Model file for the job. Use its own axes, mm. Coordinates: 2 decimals unless noted, no trailing zeros. Order: outer loops, then holes, each group sorted by start corner. A loop starts at its lowest first (then second) coordinate and runs counter-clockwise, first axis right, second up. Notation, with made-up numbers: (28, 9.5) -> (79, 9.5) arc R26 ccw to (79, 35.5) -> close; hole circle Ø1 at (-9, 2.5). An arc over 180 degrees is marked (long way). Use CSV: the item, a comma, the result in double quotes. Start each with the question number.
(1) Cut at A-A on y = -17.15. Write the cut outline in (x, z).
(2) Cut at C-C on y = -87. Write the cut outline in (x, z).
(3) Probe L1, parallel to Z at x = -3.7, y = 69.5; L2, parallel to Y at x = -2.2, z = 27; L3, parallel to Z at x = -2.2, y = -94.5. List the from-to ranges inside material, lowest first.
(4) Cut at B-B on x = -0.8. Give the number of separate pieces and of enclosed holes in the cut face, plus the area to 3 significant figures.
(5) Pin check, flat tips, straight feed: pin 1 Ø1.4 at (x, z) = (-3, 56) entering from -Y; pin 2 Ø1.4 at (x, z) = (-1.5, 55) entering from -Y. Stop position of each tip, or through.
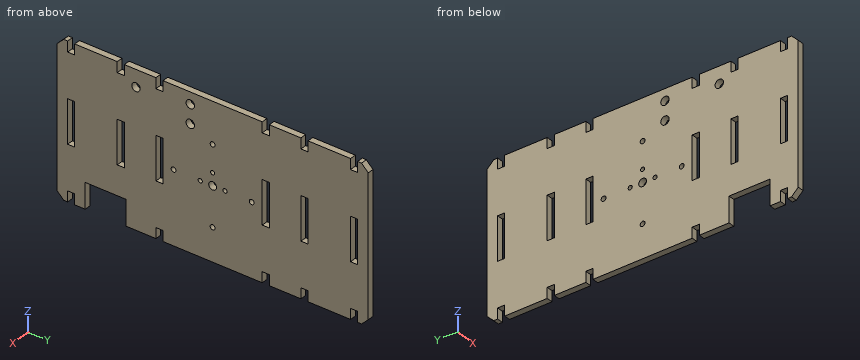
```python
from build123d import *

# Parameters (mm, degrees)
SKETCH1_R           = 1.5875
SKETCH1_R_2         = 3
SKETCH1_R_3         = 3.2385
SKETCH1_R_4         = 1.8669
SKETCH1_W           = 33.02
SKETCH1_H           = 5.461
BOSS_EXTRUDE1_DEPTH = 4.7625
CHAMFER1_SIZE       = 5.08


with BuildPart() as part:
    # Sketch1 → Boss-Extrude1 (new body)
    with BuildSketch(Plane(origin=(0, 0, 0), x_dir=(0, 0, -1), z_dir=(1, 0, 0))):
        Polygon((-58.293, 119.489), (58.293, 119.489), (58.293, 111.361), (50.293, 111.361), (50.293, 105.9), (58.293, 105.9), (58.293, 73.261), (50.293, 73.261), (50.293, 67.8), (58.293, 67.8), (58.293, 43.561), (50.293, 43.561), (50.293, 38.1), (58.293, 38.1), (58.293, -38.1), (50.293, -38.1), (50.293, -43.561), (58.293, -43.561), (58.293, -66.374), (38.857, -66.374), (38.857, -97.87), (58.293, -97.87), (58.293, -105.9), (50.293, -105.9), (50.293, -111.361), (58.293, -111.361), (58.293, -119.489), (-58.293, -119.489), (-58.293, -111.361), (-50.293, -111.361), (-50.293, -105.9), (-58.293, -105.9), (-58.293, -73.261), (-50.293, -73.261), (-50.293, -67.8), (-58.293, -67.8), (-58.293, -43.561), (-50.293, -43.561), (-50.293, -38.1), (-58.293, -38.1), (-58.293, 38.1), (-50.293, 38.1), (-50.293, 43.561), (-58.293, 43.561), (-58.293, 67.8), (-50.293, 67.8), (-50.293, 73.261), (-58.293, 73.261), (-58.293, 105.9), (-50.293, 105.9), (-50.293, 111.361), (-58.293, 111.361), align=None)
        with Locations((3, 9.519071488)):
            Circle(SKETCH1_R, mode=Mode.SUBTRACT)
        with Locations((-6.519071488, 0)):
            Circle(SKETCH1_R, mode=Mode.SUBTRACT)
        with Locations((3, -9.519071488)):
            Circle(SKETCH1_R, mode=Mode.SUBTRACT)
        with Locations((3, 0)):
            Circle(SKETCH1_R_2, mode=Mode.SUBTRACT)
        with Locations((-35.174, -17.15)):
            Circle(SKETCH1_R_3, mode=Mode.SUBTRACT)
        with Locations((-49.398, -17.15)):
            Circle(SKETCH1_R_3, mode=Mode.SUBTRACT)
        with Locations((-45.464, -58.872973782)):
            Circle(SKETCH1_R_3, mode=Mode.SUBTRACT)
        with Locations((33, 0)):
            Circle(SKETCH1_R_4, mode=Mode.SUBTRACT)
        with Locations((3, 30)):
            Circle(SKETCH1_R_4, mode=Mode.SUBTRACT)
        with Locations((-27, 0)):
            Circle(SKETCH1_R_4, mode=Mode.SUBTRACT)
        with Locations((3, -30)):
            Circle(SKETCH1_R_4, mode=Mode.SUBTRACT)
        with Locations((0, 108.6305)):
            Rectangle(SKETCH1_W, SKETCH1_H, mode=Mode.SUBTRACT)
        with Locations((0, 70.5305)):
            Rectangle(SKETCH1_W, SKETCH1_H, mode=Mode.SUBTRACT)
        with Locations((0, 40.8305)):
            Rectangle(SKETCH1_W, SKETCH1_H, mode=Mode.SUBTRACT)
        with Locations((0, -40.8305)):
            Rectangle(SKETCH1_W, SKETCH1_H, mode=Mode.SUBTRACT)
        with Locations((0, -70.5305)):
            Rectangle(SKETCH1_W, SKETCH1_H, mode=Mode.SUBTRACT)
        with Locations((0, -108.6305)):
            Rectangle(SKETCH1_W, SKETCH1_H, mode=Mode.SUBTRACT)
    extrude(amount=-BOSS_EXTRUDE1_DEPTH)

    # Chamfer1
    chamfer1_edges = [part.edges().sort_by_distance(p)[0] for p in [
        (-2.38125, 119.489, 58.293),
        (-2.38125, 119.489, -58.293),
        (-2.38125, -119.489, -58.293),
        (-2.38125, -119.489, 58.293),
    ]]
    chamfer(chamfer1_edges, length=CHAMFER1_SIZE)


solid = part.part
```
Outcome:
1,outline,"(-4.76, -58.29) -> (0, -58.29) -> (0, 31.94) -> (-4.76, 31.94) -> close; (-4.76, 38.41) -> (0, 38.41) -> (0, 46.16) -> (-4.76, 46.16) -> close; (-4.76, 52.64) -> (0, 52.64) -> (0, 58.29) -> (-4.76, 58.29) -> close"
2,outline,"(-4.76, -38.86) -> (0, -38.86) -> (0, 58.29) -> (-4.76, 58.29) -> close"
3,L1,"-50.29 to -16.51, 16.51 to 50.29"
3,L2,"-119.49 to -1.87, 1.87 to 119.49"
3,L3,"-38.86 to 58.29"
4,separate pieces,"1"
4,enclosed holes,"17"
4,area,"25,400 mm2"
5,pin 1,"y = -117.4"
5,pin 2,"y = -118.4"
